Part model, mm, in its own coordinate system. Face numbers are marked on the shaded views. A direction names the side the tool comes from. Give positions to 0.01 mm unless a question says otherwise; leave off trailing zeros. Write each loop counter-clockwise with the first axis right and the second up, starting at its lowest first coordinate (ties: lowest second). Pieces come first, ordered by that corner, then holes. Notation, with made-up numbers: M -11.5,-33 L 44.5,-33 A7 ccw 44.5,-28 Z; hole C 29,64 d11. An arc over 180 degrees is marked long. Use CSV: the item, a comma, the result in double quotes. Start each with the question number.
Item 1: Cut at D-D (y = 10.5). List the corners of the cut face in (x, z).
Item 2: Drill centre lines: line 1 (X direction, y = -20.5, z = 9.5); line 2 (Y direction, x = -21, z = 6.5); line 3 (Z direction, x = 15, y = 11). Where is each one in solid material? Low to high. Write a range as [from, to].
Item 3: Cut at C-C (x = 0.5). List the corners of the cut face in (y, z), then the cut area to 3 significant figures.
Item 4: Cut at B-B (y = -29.5). List the corners of the cut face in (x, z).
Item 5: Cut at A-A (z = 8.75). List the corners of the cut face in (x, y), then the cut area to 3 significant figures.
Item 6: Mould opens along X. For the marked faces 3, 4 and 5 say: released by +X, released by -X, zero draft, split by the parting line, or undercut.
Item 7: Which spindle directions (+Z, -Z, +X, -X, +Y, -Y) get a long thin tool onto all of the face, cutting with end or side? Do the marked faces 1 and 2. Say none if no direction does.
Item 8: Pin check, flat tips, straight feed: pin 1 (8 mm diameter, centred on x = 6.5, y = -25, fed in from +Z); pin 2 (18 mm diameter, centred on x = -3.5, y = -7.5, fed in from +Z). Stop position of each tip, or through.
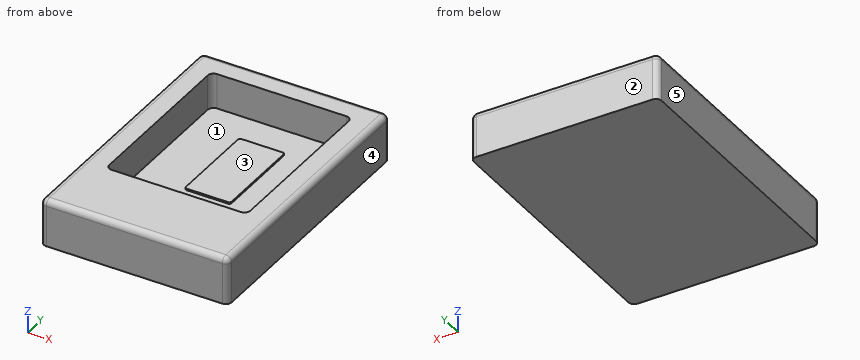
from build123d import *

# Parameters (mm, degrees)
F0_W     = 80.2
F0_H     = 115.2
F0_W_2   = 60.2
F0_H_2   = 75.2
F1_DEPTH = 20
F0_W_3   = 19.5
F0_H_3   = 39
F2_DEPTH = 5
F3_R     = 2.5
F4_R     = 2.5
F5_DEPTH = 5.7
F6_R     = 1


with BuildPart() as f1:
    # F0 (on Top) → F1 (new body)
    with BuildSketch(Plane.XY):
        with Locations((0, -10)):
            Rectangle(F0_W, F0_H)
        Rectangle(F0_W_2, F0_H_2, mode=Mode.SUBTRACT)
    extrude(amount=F1_DEPTH)

    # F0 (on Top) → F2 (join)
    with BuildSketch(Plane.XY):
        Rectangle(F0_W_2, F0_H_2)
        with Locations((0, 4.1)):
            Rectangle(F0_W_3, F0_H_3, mode=Mode.SUBTRACT)
    extrude(amount=F2_DEPTH)

    # F3
    f3_edges = [f1.edges().sort_by_distance(p)[0] for p in [
        (-30.1, 37.6, 12.5),
        (30.1, 37.6, 12.5),
        (-30.1, -37.6, 12.5),
        (30.1, -37.6, 12.5),
    ]]
    fillet(f3_edges, radius=F3_R)

    # F4
    f4_edges = [f1.edges().sort_by_distance(p)[0] for p in [
        (-40.1, -67.6, 10),
        (40.1, -67.6, 10),
        (40.1, 47.6, 10),
        (-40.1, 47.6, 10),
        (40.1, -10, 20),
        (0, -67.6, 20),
        (0, 47.6, 20),
        (-40.1, -10, 20),
    ]]
    fillet(f4_edges, radius=F4_R)

    # F0 (on Top) → F5 (join)
    with BuildSketch(Plane.XY):
        with Locations((0, 4.1)):
            Rectangle(F0_W_3, F0_H_3)
    extrude(amount=F5_DEPTH)

    # F6
    f6_edges = [f1.edges().sort_by_distance(p)[0] for p in [
        (-9.75, -15.4, 5.35),
        (9.75, -15.4, 5.35),
        (9.75, 23.6, 5.35),
        (-9.75, 23.6, 5.35),
    ]]
    fillet(f6_edges, radius=F6_R)


solid = f1.part
Worked answers:
1,outline,"M -40.1,0 L 40.1,0 L 40.1,17.5 A2.5 ccw 37.6,20 L 30.1,20 L 30.1,5 L 9.75,5 L 9.75,5.7 L -9.75,5.7 L -9.75,5 L -30.1,5 L -30.1,20 L -37.6,20 A2.5 ccw -40.1,17.5 Z"
2,line 1,"x = [-40.1, -30.1], [30.1, 40.1]"
2,line 2,"y = [-67.6, -37.6], [37.6, 47.6]"
2,line 3,"z = [0, 5]"
3,outline,"M -67.6,0 L 47.6,0 L 47.6,17.5 A2.5 ccw 45.1,20 L 37.6,20 L 37.6,5 L 23.6,5 L 23.6,5.7 L -15.4,5.7 L -15.4,5 L -37.6,5 L -37.6,20 L -65.1,20 A2.5 ccw -67.6,17.5 Z"
3,area,"1,200 mm^2"
4,outline,"M -40.1,0 L 40.1,0 L 40.1,17.5 A2.5 ccw 37.6,20 L 30.1,20 L 30.1,5 L -30.1,5 L -30.1,20 L -37.6,20 A2.5 ccw -40.1,17.5 Z"
5,outline,"M -40.1,-65.1 A2.5 ccw -37.6,-67.6 L 37.6,-67.6 A2.5 ccw 40.1,-65.1 L 40.1,45.1 A2.5 ccw 37.6,47.6 L -37.6,47.6 A2.5 ccw -40.1,45.1 Z; hole M -30.1,-35.1 A2.5 ccw -27.6,-37.6 L 27.6,-37.6 A2.5 ccw 30.1,-35.1 L 30.1,35.1 A2.5 ccw 27.6,37.6 L -27.6,37.6 A2.5 ccw -30.1,35.1 Z"
5,area,"4,710 mm^2"
6,face 3,"undercut"
6,face 4,"released by +X"
6,face 5,"released by -X"
7,face 1,"+Z"
7,face 2,"+Z, -Z, +X, -X, +Y"
8,pin 1,"stops at z = 5"
8,pin 2,"stops at z = 5.7"
